```python
from build123d import *
from build123d.topology import SkipClean

# Parameters (mm, degrees)
SKETCH1_R               = 3.2639
BOSS_EXTRUDE1_DEPTH     = 6.35
FILLET1_R               = 6.35
SKETCH6_R               = 3.2639
CUT_EXTRUDE1_DEPTH      = 246.360186308
CUT_EXTRUDE2_START      = -0.79375
CUT_EXTRUDE2_DEPTH      = 10.82675
CIRPATTERN1_COUNT       = 4
CIRPATTERN1_ANGLE       = 33
BOSS_EXTRUDE2_DEPTH     = 6.35
CUT_EXTRUDE3_DEPTH      = 251.739762675
CUT_EXTRUDE3_DEPTH_BACK = 251.739762675
SKETCH9_R               = 3.2639
FILLET2_R               = 7.9375


with BuildPart() as part:
    # Sketch1 → Boss-Extrude1 (new body)
    with BuildSketch(Plane(origin=(0, 0, 0), x_dir=(0, 0, -1), z_dir=(1, 0, 0))):
        with BuildLine():
            Line((152.4, 0), (152.4, -50.8))
            Line((152.4, -50.8), (203.2, -50.8))
            Line((203.2, -50.8), (203.2, 0))
            ThreePointArc((203.2, 0), (190.945540544, 69.498493124), (155.660230842, 130.614442288))
            Line((155.660230842, 130.614442288), (143.955847531, 137.371971144))
            Line((143.955847531, 137.371971144), (119.633936462, 116.963464536))
            Line((119.633936462, 116.963464536), (116.745173131, 97.960831716))
            ThreePointArc((116.745173131, 97.960831716), (143.209155408, 52.123869843), (152.4, 0))
        make_face()
        with Locations((165.1, -38.1)):
            Circle(SKETCH1_R, mode=Mode.SUBTRACT)
        with Locations((190.5, -38.1)):
            Circle(SKETCH1_R, mode=Mode.SUBTRACT)
    extrude(amount=BOSS_EXTRUDE1_DEPTH)

    # Sketch2 → Cut-Revolve2 (revolve, cut)
    with SkipClean():  # the faces are left unmerged after this step: merging them gives an invalid solid
        with BuildSketch(Plane(origin=(0, 0, 0), x_dir=(1, 0, 0), z_dir=(0, 1, 0))):
            with BuildLine():
                Line((-143.256, 38.1), (-25.4, 38.1))
                Line((-25.4, 38.1), (92.456, 38.1))
                ThreePointArc((92.456, 38.1), (-25.4, 155.956), (-143.256, 38.1))
            make_face()
        revolve(axis=Axis((0, 0, 0), (-1, 0, 0)), mode=Mode.SUBTRACT)
    add(part.part.scale(1), mode=Mode.REPLACE)  # the faces are merged on a copy

    # Fillet1
    fillet1_edges = [part.edges().sort_by_distance(p)[0] for p in [
        (4.841164554, 97.960831716, -116.745173131),
        (3.175, 116.963464536, -119.633936462),
        (3.175, 130.614442288, -155.660230842),
        (1.671163996, 98.49343633, -116.826139211),
    ]]
    fillet(fillet1_edges, radius=FILLET1_R)

    # Sketch6 → Cut-Extrude1 (cut, through all)
    with BuildSketch(Plane(origin=(6.35, 0, 0), x_dir=(0, 0, -1), z_dir=(1, 0, 0))):
        with Locations((167.634662821, 14.666132611)):
            Circle(SKETCH6_R)
        with Locations((192.938008153, 16.879888477)):
            Circle(SKETCH6_R)
        with Locations((161.756311884, 46.38287605)):
            Circle(SKETCH6_R)
        with Locations((186.172358961, 53.384064888)):
            Circle(SKETCH6_R)
        with Locations((149.934122858, 76.395251344)):
            Circle(SKETCH6_R)
        with Locations((172.565688572, 87.926610037)):
            Circle(SKETCH6_R)
        with Locations((132.602509563, 103.60043476)):
            Circle(SKETCH6_R)
        with Locations((152.617982705, 119.238236234)):
            Circle(SKETCH6_R)
        with BuildLine():
            Line((167.676482547, 57.989309797), (172.927374175, 39.67727449))
            ThreePointArc((172.927374175, 39.67727449), (177.639959562, 37.065045754), (180.252188298, 41.777631141))
            Line((180.252188298, 41.777631141), (175.00129667, 60.089666448))
            ThreePointArc((175.00129667, 60.089666448), (170.288711283, 62.701895184), (167.676482547, 57.989309797))
        make_face()
        with BuildLine():
            Line((153.530911348, 88.918064029), (162.179430368, 71.944389743))
            ThreePointArc((162.179430368, 71.944389743), (167.303869029, 70.27935869), (168.968900082, 75.403797351))
            Line((168.968900082, 75.403797351), (160.320381062, 92.377471637))
            ThreePointArc((160.320381062, 92.377471637), (155.195942401, 94.04250269), (153.530911348, 88.918064029))
        make_face()
        with BuildLine():
            Line((175.660675238, 24.929701663), (177.320992137, 5.952192665))
            ThreePointArc((177.320992137, 5.952192665), (181.448557317, 2.488754245), (184.911995737, 6.616319424))
            Line((184.911995737, 6.616319424), (183.251678837, 25.593828423))
            ThreePointArc((183.251678837, 25.593828423), (179.124113658, 29.057266843), (175.660675238, 24.929701663))
        make_face()
        with BuildLine():
            Line((139.748391553, 121.270808146), (151.476742658, 106.25920329))
            ThreePointArc((151.476742658, 106.25920329), (150.820091907, 100.911212098), (145.472100715, 101.567862848))
            Line((145.472100715, 101.567862848), (133.74374961, 116.579467704))
            ThreePointArc((133.74374961, 116.579467704), (134.400400361, 121.927458896), (139.748391553, 121.270808146))
        make_face()
    extrude(amount=-CUT_EXTRUDE1_DEPTH, mode=Mode.SUBTRACT)

    # Sketch8 → Cut-Extrude2 (cut)
    with BuildSketch(Plane(origin=(6.35, 15.551634957, -177.756000954), x_dir=(0, 0.08715574274765883, -0.9961946980917454), z_dir=(1, 0, 0)).offset(CUT_EXTRUDE2_START)):
        with BuildLine():
            Line((6.35, 3.175), (-1.27, 3.175))
            ThreePointArc((-1.27, 3.175), (-4.445, 0), (-1.27, -3.175))
            Line((-1.27, -3.175), (6.35, -3.175))
            ThreePointArc((6.35, -3.175), (9.525, 0), (6.35, 3.175))
        make_face()
    cut_extrude2 = extrude(amount=CUT_EXTRUDE2_DEPTH, mode=Mode.SUBTRACT)

    # CirPattern1: Cut-Extrude2 ×4 about axis
    cirpattern1_axis = Axis((0, 0, 0), (1, 0, 0))
    for i in range(1, CIRPATTERN1_COUNT):
        add(cut_extrude2.rotate(cirpattern1_axis, i * CIRPATTERN1_ANGLE / (CIRPATTERN1_COUNT - 1)), mode=Mode.SUBTRACT)

    # Sketch11 → Boss-Extrude2 (add)
    with BuildSketch(Plane(origin=(6.35, 0, 0), x_dir=(0, 0, -1), z_dir=(1, 0, 0))):
        with BuildLine():
            Line((164.098538098, 146.764662011), (143.955847531, 137.371971144))
            Line((143.955847531, 137.371971144), (154.682623198, 131.178864325))
            ThreePointArc((154.682623198, 131.178864325), (155.603036102, 130.532446831), (156.394965882, 129.733783753))
            ThreePointArc((156.394965882, 129.733783753), (165.779619803, 117.504713343), (174.21022582, 104.599413095))
            Line((174.21022582, 104.599413095), (177.102576801, 137.659136084))
            Line((177.102576801, 137.659136084), (164.098538098, 146.764662011))
        make_face()
    extrude(amount=-BOSS_EXTRUDE2_DEPTH)

    # Sketch9 → Cut-Extrude3 (cut, two sides: drawn at the far end of the back side and taken through both)
    with BuildSketch(Plane(origin=(6.35, 0, 0), x_dir=(0, 0, -1), z_dir=(1, 0, 0)).offset(-CUT_EXTRUDE3_DEPTH_BACK)):
        with Locations((168.77278845, 136.669509324)):
            Circle(SKETCH9_R)
    extrude(amount=CUT_EXTRUDE3_DEPTH + CUT_EXTRUDE3_DEPTH_BACK, mode=Mode.SUBTRACT)

    # Fillet2
    fillet2_edges = [part.edges().sort_by_distance(p)[0] for p in [
        (3.175, 146.764662011, -164.098538098),
        (3.175, 137.659136084, -177.102576801),
        (3.175, 104.599413095, -174.21022582),
    ]]
    fillet(fillet2_edges, radius=FILLET2_R)


solid = part.part
```
Geometry check sheet. Reference: the model listing, model coordinates, mm. A direction names the side the tool comes from. Give positions to 0.01 mm unless a question says otherwise; leave off trailing zeros. Loops run counter-clockwise (first coordinate to the right, second up) from the corner with the lowest first, then second, coordinate; pieces in that order, holes last. Notation, with made-up numbers: M -31.75,35 L -2.75,35 A25 ccw -2.75,65 Z; hole C 47.25,4.25 d1. An arc over 180 degrees is marked long. Write item = value, one per line. Start each with the question number.
1. Section check A-A, the plane y = -38.1. Enter the section's corners in (x, z), plus the area to 3 significant figures.
2. Tool access check on faces 1 (the face through (3.219, 142.185, -170.639)), 2 (the face through (5.556, 49, -169)), 3 (the face through (3.22, 108.97, -139.69)). Record the directions out of +Z, -Z, +X, -X, +Y, -Y that give a thin tool (end or side, any length) a straight path to the whole face; none if there is none.
3. Go/stop test with flat-tipped pins: P1, Ø2, axis at x = 3.5, y = 38.5, coming from the -Z side; P2, Ø4, axis at y = -38.1, z = -190.5, coming from the -X side; P3, Ø1.4, axis at y = 80.5, z = -157.5, coming from the +X side. Record where each tip stops, or that it passes through.
4. Draft check along Z on faces 4 (the face through (3.131, 104.745, -174.587)), 5 (the face through (3.219, 52.134, -189.187)), 6 (the face through (3, -50.8, -177)). Enter one of: +Z half, -Z half, draft (parallel to the pull), parting line (faces both ways), or undercut.
5. Thickness scan on probe 1 along Z at (x, y) = (3, 13.5); probe 2 along Y at (x, z) = (3, -135); probe 3 along Z at (x, y) = (3, 104.5). Record the ranges inside material, lowest first.
6. Section check B-B, the plane x = 2.25. Give the number of separate pieces and of enclosed holes in the cut face, plus the area to 3 significant figures.
Values follow:
q1.outline = M 0,-203.2 L 6.35,-203.2 L 6.35,-193.76 L 0,-193.76 Z; M 0,-187.24 L 6.35,-187.24 L 6.35,-168.36 L 0,-168.36 Z; M 0,-161.84 L 6.35,-161.84 L 6.35,-152.4 L 0,-152.4 Z
q1.area = 240 mm^2
q2.face_1 = -Z, +X, -X, +Y
q2.face_2 = +X
q2.face_3 = +X, -X
q3.P1 = -199.71
q3.P2 = through
q3.P3 = 5.56
q4.face_4 = -Z half
q4.face_5 = undercut
q4.face_6 = draft
q5.probe_1 = -202.75 to -184.31, -176.66 to -170.68, -164.59 to -151.88
q5.probe_2 = 70.89 to 101.39, 105.82 to 114.97, 122.31 to 129.86
q5.probe_3 = -174.65 to -152.24, -143.18 to -135.74, -129.47 to -117.74
q6.separate_pieces = 1
q6.enclosed_holes = 15
q6.area = 8,840 mm^2
